Part model, mm, in its own coordinate system. Round coordinates to 2 decimals unless told otherwise and drop trailing zeros. Loops run counter-clockwise (first coordinate to the right, second up) from the corner with the lowest first, then second, coordinate; pieces in that order, holes last.
Autodesk Inventor part; units mm, degrees
ref_plane "YZ Plane" through (0, 0, 0) normal (1, 0, 0) x (0, 1, 0)
ref_plane "XZ Plane" through (0, 0, 0) normal (0, 1, 0) x (-1, 0, 0)
ref_plane "XY Plane" through (0, 0, 0) normal (0, 0, 1) x (1, 0, 0)
sketch "Boceto1" plane through (0, 0, 0) normal (0, 0, 1) x (1, 0, 0)
  line L0 (0, 65) -> (-3, 65)
  line L1 (-3, 65) -> (-3, 15)
  line L2 (-3, 15) -> (0, 15)
  line L3 (0, 0) -> (0, 15)
  line L4 (0, 65) -> (0, 100)
  line L5 (194, 65) -> (197, 65)
  line L6 (197, 65) -> (197, 15)
  line L7 (197, 15) -> (194, 15)
  line L8 (194, 100) -> (194, 65)
  line L9 (194, 15) -> (194, 0)
  line L10 (15, 0) -> (15, 65)
  line L11 (15, 65) -> (50, 65)
  line L12 (50, 65) -> (50, 0)
  line L13 (15, 0) -> (0, 0)
  line L14 (113.5, 0) -> (113.5, 65)
  line L15 (113.5, 65) -> (148.5, 65)
  line L16 (148.5, 65) -> (148.5, 0)
  line L17 (194, 0) -> (148.5, 0)
  line L18 (95.5, 55) -> (98.5, 55)
  line L19 (98.5, 55) -> (98.5, 25)
  line L20 (98.5, 25) -> (95.5, 25)
  line L21 (95.5, 25) -> (95.5, 55)
  line L22 (59, 100) -> (59, 103)
  line L23 (59, 103) -> (109, 103)
  line L24 (109, 103) -> (109, 100)
  line L25 (0, 100) -> (59, 100)
  line L26 (109, 100) -> (194, 100)
  line L27 (109, 100) -> (209, 100) construction
  line L28 (59, 0) -> (59, -3)
  line L29 (59, -3) -> (109, -3)
  line L30 (109, -3) -> (109, 0)
  line L31 (113.5, 0) -> (109, 0)
  line L32 (59, 0) -> (50, 0)
  dimension "d0" = 194
  dimension "d1" = 100
  dimension "d3" = 50
  dimension "d8" = 3
  dimension "d13" = 35
  dimension "d14" = 65
  dimension "d15" = 15
  dimension "d16" = 3
  dimension "d17" = 30
  dimension "d19" = 95.5
  dimension "d20" = 15
  dimension "d23" = 15
  dimension "d24" = 3
  dimension "d25" = 50
  dimension "d26" = 88
  dimension "d28" = 3
  dimension "d29" = 25
extrude "Extrusión1" add sketch "Boceto1" along normal blind 3
sketch "Boceto3" plane through (0, 0, 3) normal (0, 0, 1) x (1, 0, 0)
  line L0 (124, 93.5) -> (144, 93.5)
  line L1 (144, 93.5) -> (144, 90.5)
  line L2 (144, 90.5) -> (124, 90.5)
  line L3 (124, 90.5) -> (124, 93.5)
  line L4 (148.5, 0) -> (194, 0)
  line L5 (194, 65) -> (194, 100)
  point P0 (0, 0)
  dimension "d44" = 20
  dimension "d45" = 3
  dimension "d46" = 90.5
  dimension "d47" = 50
extrude "Extrusión4" cut sketch "Boceto3" against normal blind 3
properties part number "Celda celdas" material "Madera (roble)"
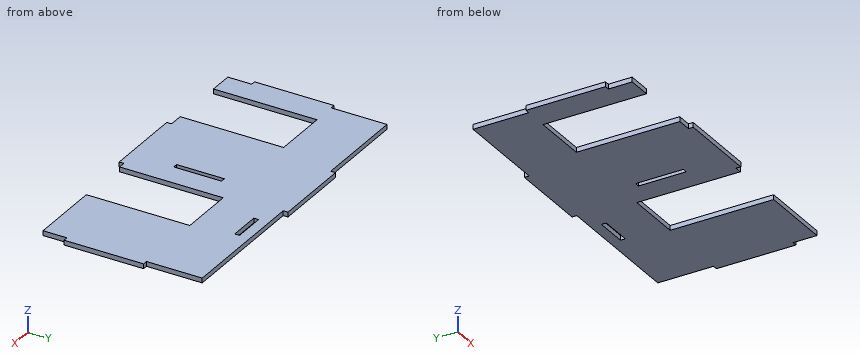
1) Slice it at D-D, the plane z = 1.2. Give the number of separate pieces and of enclosed holes in the cut face, then the cut area to 3 significant figures.
Values:
separate pieces: 1
enclosed holes: 2
area: 15,300 mm2
2) Wall check: line 1 along X through (y, z) = (49, 1.4); line 2 along X through (y, z) = (56, 0.3); line 3 along X through (y, z) = (6, 0.95). Give the ranges that are in metal, low to high.
Values:
line 1: x = -3 to 15, 50 to 95.5, 98.5 to 113.5, 148.5 to 197
line 2: x = -3 to 15, 50 to 113.5, 148.5 to 197
line 3: x = 0 to 15, 50 to 113.5, 148.5 to 194
3) Slice it at A-A, the plane y = 17. Give the cut face in (x, z).
Values:
outline: (-3, 0) - (15, 0) - (15, 3) - (-3, 3) - close; (50, 0) - (113.5, 0) - (113.5, 3) - (50, 3) - close; (148.5, 0) - (197, 0) - (197, 3) - (148.5, 3) - close
4) Slice it at C-C, the plane x = 26. Give the cut face in (y, z).
Values:
outline: (65, 0) - (100, 0) - (100, 3) - (65, 3) - close
5) Slice it at B-B, the plane y = 32.5. Give the cut face in (x, z), then the cut area to 3 significant figures.
Values:
outline: (-3, 0) - (15, 0) - (15, 3) - (-3, 3) - close; (50, 0) - (95.5, 0) - (95.5, 3) - (50, 3) - close; (98.5, 0) - (113.5, 0) - (113.5, 3) - (98.5, 3) - close; (148.5, 0) - (197, 0) - (197, 3) - (148.5, 3) - close
area: 381 mm2
6) Drop flat-ended pins along their axis: pin 1 Ø0.9 at (x, z) = (137, 1) entering from -Y; pin 2 Ø1.5 at (y, z) = (101.5, 1.5) entering from +X; pin 3 Ø1.5 at (x, z) = (175, 2) entering from -Y. Give the stop position or say it passes through.
Values:
pin 1: stops at y = 65
pin 2: stops at x = 109
pin 3: stops at y = 0
